Read the model definition and answer for the solid it produces. Units are mm, in the model's axes. A direction names the side the tool comes from. Coordinates: 2 decimals unless noted, no trailing zeros. Write each loop counter-clockwise with the first axis right and the second up, starting at its lowest first coordinate (ties: lowest second). Pieces come first, ordered by that corner, then holes.
1) This flat-tipped pin is pushed along its axis until it touches: pin 1 Ø10 at (x, z) = (28, 22.5) entering from -Y. Where does it stop, or does it pass through?
2) The part is cut by section B-B (z = -4.5). Determine the outline of the cut face in (x, y), then the cut area to 3 significant figures.
3) The part is cut by section A-A (x = -29). Determine the outline of the cut face in (y, z).
4) Which of the six approach directions +Z, -Z, +X, -X, +Y, -Y give full straight-line access (tool end or side, diameter ignored) to faces 1 (the face through (62, 0, 32)), 2 (the face through (-62, 0, -32)), 3 (the face through (-62, -2, 31))?
5) Find the intervals of material crossed by line 1 (Y direction, x = 17.5, z = 6.5), in increasing order.
Autodesk Inventor part; units mm, degrees
ref_plane "YZ Plane" through (0, 0, 0) normal (1, 0, 0) x (0, 1, 0)
ref_plane "XZ Plane" through (0, 0, 0) normal (0, 1, 0) x (-1, 0, 0)
ref_plane "XY Plane" through (0, 0, 0) normal (0, 0, 1) x (1, 0, 0)
sketch "Szkic1" plane through (0, 0, 0) normal (0, 1, 0) x (-1, 0, 0)
  line L0 (63, -33) -> (-63, -33)
  line L1 (-63, -33) -> (-63, 33)
  line L2 (-63, 33) -> (63, 33)
  line L3 (63, 33) -> (63, -33)
  line L4 (63, -33) -> (-63, 33) construction
  line L5 (-63, -33) -> (63, 33) construction
  point P0 (0, 0)
  dimension "d0" = 126
  dimension "d1" = 66
extrude "Wyciągnięcie proste1" add sketch "Szkic1" along normal blind 42
sketch "Szkic2" plane through (0, 0, 0) normal (0, -1, 0) x (1, 0, 0)
  line L0 (-63, -33) -> (63, -33)
  line L1 (63, -33) -> (63, 33)
  line L2 (63, 33) -> (-63, 33)
  line L3 (-63, 33) -> (-63, -33)
  line L4 (-58, 28) -> (58, 28)
  line L5 (58, 28) -> (58, -28)
  line L6 (58, -28) -> (-58, -28)
  line L7 (-58, -28) -> (-58, 28)
  circle A0 centre (-58, 28) radius 5
  circle A1 centre (58, 28) radius 5
  circle A2 centre (58, -28) radius 5
  circle A3 centre (-58, -28) radius 5
  point P0 (0, 0)
  dimension "d4" = 5
  dimension "d5" = 10
  dimension "d6" = 10
  dimension "d7" = 10
  dimension "d8" = 10
extrude "Wyciągnięcie proste2" add sketch "Szkic2" along normal blind 5 contours A3 L7 L6 | A2 L6 L5 | L6 L7 A3 | A0 L4 L7 | A2 L5 L6 | L7 L4 A0 | A1 L5 L4 | A1 L4 L5
equation "\"d5\" = 2 * d4"
equation "\"d6\" = 2 * d4"
equation "\"d7\" = 2 * d4"
equation "\"d8\" = 2 * d4"
equation "\"d9\" = d4"
properties part number "czujnik"
Reported:
1. pin 1: stops at y = 0
2. outline: (-63, 0) - (63, 0) - (63, 42) - (-63, 42) - close
2. area: 5,290 mm2
3. outline: (0, -33) - (42, -33) - (42, 33) - (0, 33) - close
4. face 1: +Z, +X, -Y
4. face 2: -Z, -X, -Y
4. face 3: -Y
5. line 1: y = 0 to 42
